from build123d import *

# Parameters (mm, degrees)
SKETCH1_W           = 115
SKETCH1_H           = 140
BOSS_EXTRUDE1_DEPTH = 2.4
CUT_EXTRUDE1_DEPTH  = 3.4
FILLET1_R           = 10
SKETCH3_W           = 2.4
SKETCH3_H           = 140
BOSS_EXTRUDE2_DEPTH = 25
FILLET2_R           = 10
SKETCH4_R           = 2.75
CUT_EXTRUDE2_DEPTH  = 116
SKETCH5_R           = 15
SKETCH5_R_2         = 2.75
CUT_EXTRUDE3_DEPTH  = 3.4


with BuildPart() as part:
    # Sketch1 → Boss-Extrude1 (new body)
    with BuildSketch(Plane(origin=(0, 0, 0), x_dir=(0, 0, -1), z_dir=(1, 0, 0))):
        with Locations((57.5, -70)):
            Rectangle(SKETCH1_W, SKETCH1_H)
    extrude(amount=BOSS_EXTRUDE1_DEPTH)

    # Sketch2 → Cut-Extrude1 (cut, through all)
    with BuildSketch(Plane(origin=(2.4, 0, 0), x_dir=(0, 0, -1), z_dir=(1, 0, 0))):
        Polygon((87, 0), (115, -30), (142.616199658, -32.505405645), (142.616199658, 14.875556406), align=None)
        Polygon((115, -110), (87, -140), (87, -152.661109726), (136.310004643, -152.661109726), align=None)
    extrude(amount=-CUT_EXTRUDE1_DEPTH, mode=Mode.SUBTRACT)

    # Fillet1
    fillet1_edges = [part.edges().sort_by_distance(p)[0] for p in [
        (1.2, 0, -87),
        (1.2, -30, -115),
        (1.2, -110, -115),
        (1.2, -140, -87),
    ]]
    fillet(fillet1_edges, radius=FILLET1_R)

    # Sketch3 → Boss-Extrude2 (add)
    with BuildSketch(Plane(origin=(2.4, 0, 0), x_dir=(0, 0, -1), z_dir=(1, 0, 0))):
        with Locations((1.2, -70)):
            Rectangle(SKETCH3_W, SKETCH3_H)
    extrude(amount=BOSS_EXTRUDE2_DEPTH)

    # Fillet2
    fillet2_edges = [part.edges().sort_by_distance(p)[0] for p in [
        (27.4, -140, -1.2),
        (27.4, 0, -1.2),
    ]]
    fillet(fillet2_edges, radius=FILLET2_R)

    # Sketch4 → Cut-Extrude2 (cut, through all)
    with BuildSketch(Plane.XY):
        with Locations((11.974983581, -70)):
            Circle(SKETCH4_R)
        with Locations((11.974983581, -25)):
            Circle(SKETCH4_R)
        with Locations((11.974983581, -115)):
            Circle(SKETCH4_R)
    extrude(amount=-CUT_EXTRUDE2_DEPTH, mode=Mode.SUBTRACT)

    # Sketch5 → Cut-Extrude3 (cut, through all)
    with BuildSketch(Plane(origin=(2.4, 0, 0), x_dir=(0, 0, -1), z_dir=(1, 0, 0))):
        with Locations((89.027947804, -43.505970801)):
            Circle(SKETCH5_R)
        with Locations((77.277947804, -23.154373812)):
            Circle(SKETCH5_R_2)
        with Locations((100.777947804, -23.154373812)):
            Circle(SKETCH5_R_2)
        with Locations((65.527947804, -43.505970801)):
            Circle(SKETCH5_R_2)
        with Locations((77.277947804, -63.85756779)):
            Circle(SKETCH5_R_2)
        with Locations((100.777947804, -63.85756779)):
            Circle(SKETCH5_R_2)
    extrude(amount=-CUT_EXTRUDE3_DEPTH, mode=Mode.SUBTRACT)


solid = part.part
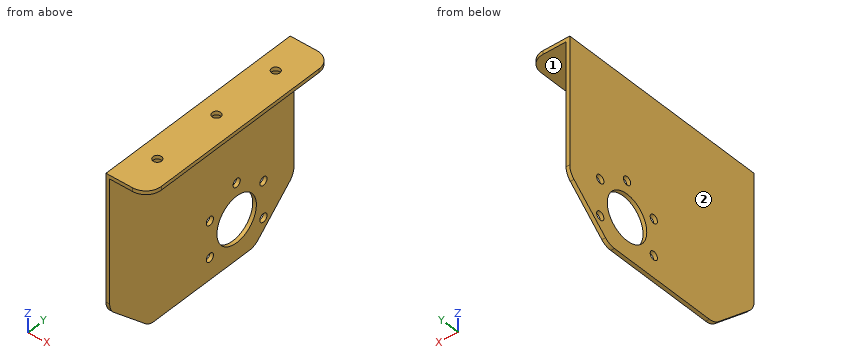
Model file for the job. Use its own axes, mm. Face numbers are marked on the shaded views. A direction names the side the tool comes from. Round coordinates to 2 decimals unless told otherwise and drop trailing zeros. Order: outer loops, then holes, each group sorted by start corner. A loop starts at its lowest first (then second) coordinate and runs counter-clockwise, first axis right, second up.
(1) Pin check, flat tips, straight feed: pin 1 (6.5 mm diameter, centred on y = -23.15, z = -77.28, fed in from +X); pin 2 (5 mm diameter, centred on x = 12.5, y = -26, fed in from -Z). Stop position of each tip, or through.
(2) Band-saw the part on D-D (y = -115). List the corners of the cut face in (x, z), then the cut area to 3 significant figures.
(3) Band-saw the part on C-C (z = -15.5). List the corners of the cut face in (x, y), then the cut area to 3 significant figures.
(4) Drill centre lines: line 1 (Z direction, x = 2, y = -41.5); line 2 (X direction, y = -76, z = -105); line 3 (Z direction, x = 25.5, y = -6.5). Where is each one in solid material? Low to high.
(5) Band-saw the part on B-B (x = 7.75). List the corners of the cut face in (y, z), then the cut area to 3 significant figures.
(6) 3-axis set-ups, long thin cutter, end or side, ignore diameter. For the marked faces 1 and 2: which of +Z, -Z, +X, -X, +Y, -Y reach the whole face in a straight line?
(7) Band-saw the part on A-A (y = -70). List the corners of the cut face in (x, z), then the cut area to 3 significant figures.
Verdict:
1. pin 1: stops at x = 2.4
1. pin 2: stops at z = -2.4
2. outline: (0, -110.33) - (2.4, -110.33) - (2.4, -2.4) - (9.22, -2.4) - (9.22, 0) - (0, 0) - close; (14.72, -2.4) - (27.4, -2.4) - (27.4, 0) - (14.72, 0) - close
2. area: 312 mm2
3. outline: (0, -140) - (2.4, -140) - (2.4, 0) - (0, 0) - close
3. area: 336 mm2
4. line 1: z = -115 to -103.89, -74.16 to -67.41, -63.65 to 0
4. line 2: x = 0 to 2.4
4. line 3: z = -2.4 to 0
5. outline: (-140, -2.4) - (0, -2.4) - (0, 0) - (-140, 0) - close
5. area: 336 mm2
6. face 1: -Z, +X, +Y, -Y
6. face 2: +Z, -Z, -X, +Y, -Y
7. outline: (0, -115) - (2.4, -115) - (2.4, -2.4) - (9.22, -2.4) - (9.22, 0) - (0, 0) - close; (14.72, -2.4) - (27.4, -2.4) - (27.4, 0) - (14.72, 0) - close
7. area: 323 mm2
